Could you check a few things on this model? Use its own coordinates, in mm. Face numbers are marked on the shaded views. A direction names the side the tool comes from. Round coordinates to 2 decimals unless told otherwise and drop trailing zeros. Write each loop counter-clockwise with the first axis right and the second up, starting at its lowest first coordinate (ties: lowest second). Pieces come first, ordered by that corner, then holes. Notation, with made-up numbers: (86.5, 7.25) - (112.5, 7.25) arc R20 ccw to (112.5, 42.25) - close; hole circle Ø10 at (84.25, 75). An arc over 180 degrees is marked (long way). Write each question's results on one line, items separated by ' | '. Start each with the question number.
(1) For P1, Ø0.7, axis at x = -0.5, y = 5.5, coming from the +Z side; P2, Ø1, axis at x = 1, y = -3, coming from the -Z side, each with a flat end and sliding along its axis, tell me the tip position at first contact or that it passes through.
(2) Imagine slicing it at C-C on y = 3.5. Write out the boundary of the cut face in (x, z), then the cut area to 3 significant figures.
(3) Please list where these lines run through material, in increasing order: line 1 (X direction, y = 4.15, z = 0.3); line 2 (Y direction, x = 0, z = 0.8); line 3 (Z direction, x = -0.55, y = 1.75). Write a range as [from, to].
(4) On a 3-axis mill with a long thin cutter (end or side, diameter ignored), from which of +Z, -Z, +X, -X, +Y, -Y can I reach the whole of each face in a straight line? I mean the marked faces 1 and 2. Say none if no direction works.
(5) Imagine slicing it at D-D on x = -1.2. Write out the boundary of the cut face in (y, z), then the cut area to 3 significant figures.
(6) Imagine slicing it at A-A on z = 0.45. Write out the boundary of the cut face in (x, y), then the cut area to 3 significant figures.
(7) Imagine slicing it at B-B on x = 0. Write out the boundary of the cut face in (y, z), then the cut area to 3 significant figures.
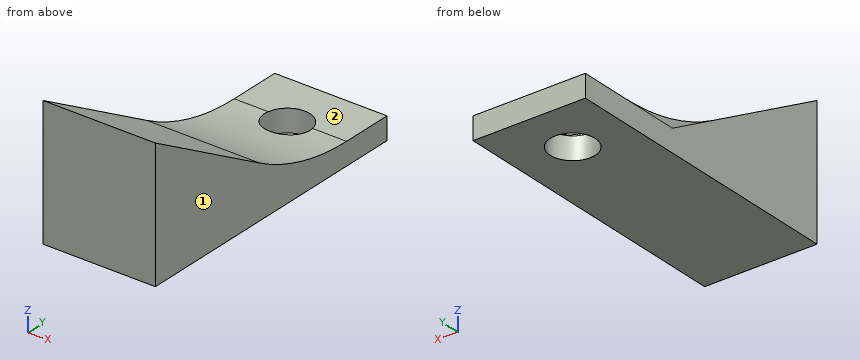
```python
from build123d import *

# Parameters (mm, degrees)
SKETCH_1_W      = 5
SKETCH_1_H      = 13.3
SKETCH_1_R      = 1
EXTRUDE_1_DEPTH = 1
EXTRUDE_3_DEPTH = 2.5
FILLET_1_R      = 10


with BuildPart() as part:
    # 草图1 → 凸台-拉伸1 (new body)
    with BuildSketch(Plane.XY):
        Rectangle(SKETCH_1_W, SKETCH_1_H)
        with Locations((0, 4.15)):
            Circle(SKETCH_1_R, mode=Mode.SUBTRACT)
    extrude(amount=EXTRUDE_1_DEPTH)

    # 草图2 → 凸台-拉伸3 (add, symmetric)
    with BuildSketch(Plane(origin=(0, 0, 0), x_dir=(0, 0, -1), z_dir=(1, 0, 0))):
        Polygon((-1, 1.65), (-5.792007234, -6.65), (-1, -6.65), align=None)
    extrude(amount=EXTRUDE_3_DEPTH, both=True)

    # 圆角1
    # the kernel refuses this fillet: 10 mm, written as the material it adds along each edge
    with BuildSketch(Plane(origin=(2.5, 1.65, 1), x_dir=(0, 1, 0), z_dir=(-1, 0, 0))) as fillet_1_piece_1_section:
        with BuildLine():
            CenterArc((FILLET_1_R * 0.267949192431, -FILLET_1_R), FILLET_1_R, 90, 30)
            Line((-FILLET_1_R * 0.232050807569, -FILLET_1_R * 0.133974596216), (0, 0))
            Line((0, 0), (FILLET_1_R * 0.267949192431, 0))
        make_face()
    fillet_1_piece_1 = extrude(amount=5, mode=Mode.PRIVATE)
    fillet_1_piece_1 = fillet_1_piece_1 - Plane(origin=(0, 4.15, 1.267699118), x_dir=(1, 0, 0), z_dir=(0, 0, -1)) * Cylinder(1, 21, mode=Mode.PRIVATE)
    add(fillet_1_piece_1)


solid = part.part
```
Response:
1) P1: z = 1 | P2: z = 0
2) outline: (-2.5, 0) - (-0.76, 0) - (-0.76, 1.03) - (-2.5, 1.03) - close; (0.76, 0) - (2.5, 0) - (2.5, 1.03) - (0.76, 1.03) - close | area: 3.60 mm²
3) line 1: [-2.5, -1], [1, 2.5] | line 2: [-6.65, 3.15], [5.15, 6.65] | line 3: [0, 1.34]
4) face 1: +Z, -Z, +X, +Y, -Y | face 2: +Z, +X, -X, +Y
5) outline: (-6.65, 0) - (6.65, 0) - (6.65, 1) - (4.33, 1) arc R10 cw to (-0.67, 2.34) - (-6.65, 5.79) - close | area: 33.8 mm²
6) outline: (-2.5, -6.65) - (2.5, -6.65) - (2.5, 6.65) - (-2.5, 6.65) - close; hole circle Ø2 at (0, 4.15) | area: 63.4 mm²
7) outline: (-6.65, 0) - (3.15, 0) - (3.15, 1.07) arc R10 cw to (-0.67, 2.34) - (-6.65, 5.79) - close; (5.15, 0) - (6.65, 0) - (6.65, 1) - (5.15, 1) - close | area: 31.8 mm²
